```python
from build123d import *

# Parameters (mm, degrees)
BOSS_EXTRU_1_DEPTH = 6.35
ESQUISSE2_W        = 6.35
ESQUISSE2_H        = 12.7
BOSS_EXTRU_2_DEPTH = 6.35


with BuildPart() as part:
    # Esquisse1 → Boss.-Extru.1 (new body)
    with BuildSketch(Plane.XY):
        Polygon((-12.7, -71.84263), (12.7, -46.44263), (12.7, 46.44263), (-12.7, 71.84263), align=None)
    extrude(amount=BOSS_EXTRU_1_DEPTH)

    # Esquisse2 → Boss.-Extru.2 (add)
    with BuildSketch(Plane(origin=(29.571315, 29.571315, 0), x_dir=(0, 0, -1), z_dir=(0.707106781186549, 0.7071067811865461, 0))):
        with Locations((-3.175, 41.784422488)):
            Rectangle(ESQUISSE2_W, ESQUISSE2_H)
    extrude(amount=BOSS_EXTRU_2_DEPTH)


solid = part.part
```
Part model, mm, in its own coordinate system. A direction names the side the tool comes from. Coordinates: 2 decimals unless noted, no trailing zeros. Write each loop counter-clockwise with the first axis right and the second up, starting at its lowest first coordinate (ties: lowest second). Pieces come first, ordered by that corner, then holes.
Item 1: Slice it at C-C (x = -6.75). Write the cut outline in (y, z).
Item 2: Mould opens along X. For faces 3 (the face through (-8.525, 67.667, 3.131)), 4 (the face through (-2.25, 65.82, 3.22)), 5 (the face through (0, 1, 6.35)), 6 (the face through (8.66, 50.48, 3.13)) say: released by +X, released by -X, zero draft, split by the parting line, or undercut.
Item 3: Which spindle directions (+Z, -Z, +X, -X, +Y, -Y) get a long thin tool onto all of the face, cutting with end or side? Do faces 1 (the face through (6.73, 56.84, 3.22)), 2 (the face through (-12.7, 1, 3)). Say none if no direction does.
Item 4: Slice it at D-D (x = 1.75). Write the cut outline in (y, z), and give its area (3 significant figures).
Item 5: Probe line 1 (X direction, y = -53, z = 4.5); line 2 (Y direction, x = 1.75, z = 4.5); line 3 (Y direction, x = -1.25, z = 1). List the from-to ranges inside material, lowest first.
Item 6: Slice it at B-B (z = 1.75). Write the cut outline in (x, y).
Item 7: Slice it at A-A (x = 7.5). Write the cut outline in (y, z).
Results found:
1. outline: (-65.89, 0) - (65.89, 0) - (65.89, 6.35) - (-65.89, 6.35) - close
2. face 3: undercut
2. face 4: undercut
2. face 5: zero draft
2. face 6: released by +X
3. face 1: +Z, -Z, +X
3. face 2: +Z, -Z, -X, +Y, -Y
4. outline: (-57.39, 0) - (66.37, 0) - (66.37, 6.35) - (-57.39, 6.35) - close
4. area: 786 mm2
5. line 1: x = -12.7 to 6.14
5. line 2: y = -57.39 to 66.37
5. line 3: y = -60.39 to 66.82
6. outline: (-12.7, -71.84) - (12.7, -46.44) - (12.7, 46.44) - (4.52, 54.63) - (9.01, 59.12) - (0.03, 68.1) - (-4.46, 63.61) - (-12.7, 71.84) - close
7. outline: (-51.64, 0) - (51.64, 0) - (51.64, 6.35) - (-51.64, 6.35) - close; (57.61, 0) - (60.62, 0) - (60.62, 6.35) - (57.61, 6.35) - close
